Autodesk Inventor part; units mm, degrees
ref_plane "to_screw1_XY" through (15, 4.2426, 4.2426) normal (0, 0.7071, 0.7071) x (1, 0, 0)
ref_plane "to_screw1_YZ" through (15, 4.2426, 4.2426) normal (1, 0, 0) x (0, 0.7071, -0.7071)
ref_plane "to_screw1_ZX" through (15, 4.2426, 4.2426) normal (0, 0.7071, -0.7071) x (0, 0.7071, 0.7071)
sketch "Sketch_1" plane through (0, 0, 0) normal (0, 0, 1) x (1, 0, 0)
  line L0 (24, 0) -> (0, 0)
  line L1 (0, 18) -> (0, 6)
  line L2 (0, 6) -> (24, 6)
  line L3 (24, 6) -> (24, 8)
  line L4 (24, 8) -> (6, 8)
  line L5 (6, 8) -> (6, 18)
  line L6 (6, 18) -> (0, 18)
revolve "Revolution1" add sketch "Sketch_1" angle 360 about axis through (24, 0, 0) along (1, 0, 0)
sketch "Sketch_3" plane through (0, 0, 0) normal (0, -0.7071, 0.7071) x (1, 0, 0)
  line L0 (15, 5.5) -> (15, 8)
  line L1 (15, 8) -> (17, 8)
  line L2 (17, 8) -> (16.621, 7.621)
  line L3 (16.621, 7.621) -> (16.621, 5.5)
  line L4 (16.621, 5.5) -> (15, 5.5)
  line L5 (15, 5.5) -> (15, 8)
revolve "Revolution2" cut sketch "Sketch_3" angle 360 about axis through (15, 3.8891, 3.8891) along (0, -0.7071, -0.7071)
thread "Thread1"
sketch "Sketch3" plane through (6, 0, 0) normal (1, 0, 0) x (0, 0, -1)
  point P0 (0, 13)
hole "Hole1" at (6, 13, 0) direction (-1, 0, 0) diameter 4.5 depth 6
sketch "Sketch4" plane through (6, 0, 0) normal (1, 0, 0) x (0, 0, -1)
  point P0 (0, -13)
hole "Hole2" at (6, -13, 0) direction (-1, 0, 0) diameter 4.5 depth 6
sketch "Sketch5" plane through (6, 0, 0) normal (1, 0, 0) x (0, 0, -1)
  point P0 (-13, 0)
hole "Hole3" at (6, 0, 13) direction (-1, 0, 0) diameter 4.5 depth 6
sketch "Sketch6" plane through (6, 0, 0) normal (1, 0, 0) x (0, 0, -1)
  point P0 (13, 0)
hole "Hole4" at (6, 0, -13) direction (-1, 0, 0) diameter 4.5 depth 6
sketch "Sketch_2" plane through (0, 0, 0) normal (0, -0.7071, -0.7071) x (1, 0, 0)
  line L0 (15, 5.5) -> (15, 8)
  line L1 (15, 8) -> (17, 8)
  line L2 (17, 8) -> (16.621, 7.621)
  line L3 (16.621, 7.621) -> (16.621, 5.5)
  line L4 (16.621, 5.5) -> (15, 5.5)
  line L5 (15, 5.5) -> (15, 8)
revolve "Revolution3" cut sketch "Sketch_2" angle 360 about axis through (15, -3.8891, 3.8891) along (0, 0.7071, -0.7071)
thread "Thread2"
ref_plane "to_screw1_XY" through (15, 4.2426, 4.2426) normal (0, 0.7071, 0.7071) x (1, 0, 0)
ref_plane "to_screw1_YZ" through (15, 4.2426, 4.2426) normal (1, 0, 0) x (0, 0.7071, -0.7071)
ref_plane "to_screw1_ZX" through (15, 4.2426, 4.2426) normal (0, 0.7071, -0.7071) x (0, 0.7071, 0.7071)
ref_plane "to_screw2_XY" through (15, -4.2426, 4.2426) normal (0, -0.7071, 0.7071) x (1, 0, 0)
ref_plane "to_screw2_YZ" through (15, -4.2426, 4.2426) normal (1, 0, 0) x (0, 0.7071, 0.7071)
ref_plane "to_screw2_ZX" through (15, -4.2426, 4.2426) normal (0, 0.7071, 0.7071) x (0, -0.7071, 0.7071)
properties part number "BTHR12-MB_b"
The model under review builds one solid part; all positions refer to its coordinate system, in mm. Give positions to 0.01 mm unless a question says otherwise; leave off trailing zeros. Order: outer loops, then holes, each group sorted by start corner. A loop starts at its lowest first (then second) coordinate and runs counter-clockwise, first axis right, second up. Notation, with made-up numbers: M 8,34 L 52,34 A19 ccw 52,46 Z; hole C 28,-22.5 d9. An arc over 180 degrees is marked long. Use one line per item in the form item = value. Start each with the question number.
Item 1: We need section C-C on x = 4.5. Give the boundary of the cut face in (y, z).
Item 2: The part is to be moulded in two halves that separate along Y. For faces 1 (the cylindrical face through (2.96, -15.23, 0.29)), 2 (the cylindrical face through (2.958, -0.099, 15.248)), 3 (the flat face through (6, 8, -4)), 4 (the cylindrical face through (14.87, 7.63, -2.4)), say which applies: pulls with the +Y half, pulls with the -Y half, needs draft (parallel to the pull), parting line crosses it, or undercut.
Item 3: We need section A-A on z = 0. Give the boundary of the cut face in (x, y).
Item 4: We need section D-D on y = 14. Give the boundary of the cut face in (x, z), plus the area to 3 significant figures.
Item 5: To check wall thickness, follow line 1 along Z through (x, y) = (2.5, 0); line 2 along X through (y, z) = (14, -5.5); line 3 along Z through (x, y) = (3.4, -13). State the ranges of each line that lie inside material, in increasing order. Write a range as from..to.
Item 6: Insertion check: pin 1 Ø9.5 at (y, z) = (0, 0) entering from -X; pin 2 Ø6 at (x, y) = (7.5, -6.5) entering from +Z; pin 3 Ø2 at (x, z) = (6, 13) entering from -Y; pin 4 Ø12 at (y, z) = (1, 14.5) entering from +X. Each pin has a flat end and moves straight along its axis. Give the tip position at first contact, or say it passes through.
Completed:
q1.outline = C 0,0 d36; hole C -13,0 d4.5; hole C 0,0 d12; hole C 0,-13 d4.5; hole C 0,13 d4.5; hole C 13,0 d4.5
q2.face_1 = undercut
q2.face_2 = undercut
q2.face_3 = needs draft
q2.face_4 = parting line crosses it
q3.outline = M 0,-18 L 6,-18 L 6,-15.25 L 0,-15.25 Z; M 0,-10.75 L 6,-10.75 L 6,-8 L 24,-8 L 24,-6 L 0,-6 Z; M 0,6 L 24,6 L 24,8 L 6,8 L 6,10.75 L 0,10.75 Z; M 0,15.25 L 6,15.25 L 6,18 L 0,18 Z
q4.outline = M 0,-11.31 L 6,-11.31 L 6,-2.02 L 0,-2.02 Z; M 0,2.02 L 6,2.02 L 6,11.31 L 0,11.31 Z
q4.area = 112 mm²
q5.line_1 = -18..-15.25, -10.75..-6, 6..10.75, 15.25..18
q5.line_2 = 0..6
q5.line_3 = -12.45..-2.25, 2.25..12.45
q6.pin_1 = through
q6.pin_2 = 17.57
q6.pin_3 = -13.42
q6.pin_4 = 6
